```python
from build123d import *

# Parameters (mm, degrees)
CUT_EXTRUDE1_DEPTH      = 14.866731381
CUT_EXTRUDE1_DEPTH_BACK = 14.866731381
SKETCH2_R               = 1.5
SCALE1_SCALE            = 1.5


with BuildPart() as part:
    # Sketch1 → Revolve1 (revolve)
    with BuildSketch(Plane.XY, mode=Mode.PRIVATE) as revolve1_sk:
        with BuildLine():
            Line((-7, 8.712098042), (-7, 7.295703465))
            Line((-7, 7.295703465), (-6, 7.295703465))
            Line((-6, 7.295703465), (-6, 6.795703465))
            Line((-6, 6.795703465), (-7, 6.795703465))
            Line((-7, 6.795703465), (-7, 6.295703465))
            Line((-7, 6.295703465), (-6, 6.295703465))
            Line((-6, 6.295703465), (-6, 5.795703465))
            Line((-6, 5.795703465), (-7, 5.795703465))
            Line((-7, 5.795703465), (-7, -5.204296535))
            Line((-7, -5.204296535), (-6.25, -5.204296535))
            Line((-6.25, -5.204296535), (-5.050561785, -1.908867124))
            ThreePointArc((-5.050561785, -1.908867124), (-4.825715591, -1.069729704), (-4.75, -0.204296535))
            Line((-4.75, -0.204296535), (-4.75, 4.440083994))
            ThreePointArc((-4.75, 4.440083994), (-4.399873792, 5.550542455), (-3.476134386, 6.259352631))
            Line((-3.476134386, 6.259352631), (0, 7.524562078))
            Line((0, 7.524562078), (0, 8.566185983))
            Line((0, 8.566185983), (0, 9.69172121))
            add(Edge.make_bspline(
                [(-7, 8.712098042), (-6.915941705, 9.672888752), (-6.571850582, 9.786532429), (-6.017076444, 9.562037769), (-5.173496459, 8.320355176), (-3.929482137, 7.778040067), (-3.257853738, 7.770566701), (-1.62159895, 8.374478133), (-0.988089519, 9.078164836), (-0.514286955, 9.634062862), (-0.187546651, 9.695286605), (0, 9.69172121)],
                knots=[0, 0, 0, 0, 0.210746943, 0.254088111, 0.413486836, 0.459298403, 0.666392212, 0.714990212, 0.896680404, 0.92745251, 1, 1, 1, 1], degree=3))
        make_face()
    revolve(revolve1_sk.sketch.rotate(Axis((0, 2.420801252, 0), (0, 1, 0)), 270), axis=Axis((0, 2.420801252, 0), (0, 1, 0)))

    # Sketch2 → Cut-Extrude1 (cut, two sides: drawn at the far end of the back side and taken through both)
    with BuildSketch(Plane.XY.offset(-CUT_EXTRUDE1_DEPTH_BACK)):
        with Locations((0, 1.795703465)):
            Circle(SKETCH2_R)
    extrude(amount=CUT_EXTRUDE1_DEPTH + CUT_EXTRUDE1_DEPTH_BACK, mode=Mode.SUBTRACT)


with BuildPart() as part_1:
    # Scale1: scaled about (1.0568e-05, 2.939086838, 0.000578627)
    add(part.part.scale(SCALE1_SCALE).moved(Location((-5.284e-06, -1.469543419, -0.000289313))))


solid = part_1.part
```
Here's how the part is built. I have some questions about the finished solid (model axes, mm). A direction names the side the tool comes from. Give positions to 0.01 mm unless a question says otherwise; leave off trailing zeros. Loops run counter-clockwise (first coordinate to the right, second up) from the corner with the lowest first, then second, coordinate; pieces in that order, holes last. Notation, with made-up numbers: M 36.5,-18 L 65.5,-18 A25 ccw 65.5,21 Z; hole C 52,41.25 d3. An arc over 180 degrees is marked long. Use one line per item in the form item = value. Start each with the question number.
Q1. Which directions (+Z, -Z, +X, -X, +Y, -Y) give clear straight access to the entire face, cutting with the end or side of a thin tool? Please do faces 1 (the flat face through (-5, 7.224, 8)), 2 (the cylindrical face through (2.146, 1.9, 8.607)).
Q2. Will these pins go through, and if not, where does the flat tip stop? pin 1 Ø10.5 at (x, z) = (4, 2.5) entering from -Y; pin 2 Ø1.5 at (y, z) = (0, -5.5) entering from +X; pin 3 Ø6 at (y, z) = (-7, -6.5) entering from -X; pin 4 Ø2 at (x, z) = (6.5, -4.5) entering from +Y.
Q3. If we section it at C-C (y = 5.5): Write out the boundary of the cut face in (x, z).
Q4. I need wall thicknesses on line 1 along Y through (x, z) = (7.75, -6); line 2 along Y through (x, z) = (-2, -9.25); line 3 along X through (y, z) = (-7.5, -1.5). Which ranges of each line are inside material? Lowest first, please.
Q5. Thinking about a two-plate mould opening in Z: for faces 3 (the conical face through (4.66, -4.57, 6.08)), 4 (the cylindrical face through (-3.2, 10.5, -10)), 5 (the flat face through (-9, -9.276, 4)), 6 (the cylindrical face through (2.73, 1.76, -6.58)), which applies, +Z half, -Z half, draft (parallel to the pull), parting line (faces both ways), or undercut?
Q6. If we section it at B-B (x = 1.25): State how many separate pieces and enclosed holes the cut face has, then the cut area to 3 significant figures.
Q7. If we section it at A-A (y = -0.25): Write out the boundary of the cut face in (x, z) (3 decimals), then the cut area to 3 significant figures.
Taken from the geometry:
q1.face_1 = none
q1.face_2 = +Z, -Z
q2.pin_1 = -9.28
q2.pin_2 = 9.36
q2.pin_3 = -9.9
q2.pin_4 = 12.57
q3.outline = C 0,0 d21; hole C 0,0 d14.22
q4.line_1 = -9.28 to 7.22, 7.97 to 8.72, 9.47 to 13.09
q4.line_2 = -9.28 to 0.19, 2.25 to 7.22, 7.97 to 8.72, 9.47 to 13.04
q4.line_3 = -10.39 to -8.6, 8.6 to 10.39
q5.face_3 = undercut
q5.face_4 = parting line
q5.face_5 = draft
q5.face_6 = undercut
q6.separate_pieces = 3
q6.enclosed_holes = 0
q6.area = 139 mm^2
q7.outline = M -1.7,-10.362 L -1.7,-6.92 A7.125 cw -1.7,6.919 L -1.7,10.361 A10.5 ccw Z; M 1.7,-10.362 A10.5 ccw 1.7,10.361 L 1.7,6.919 A7.125 cw 1.7,-6.92 Z
q7.area = 164 mm^2
